The model under review builds one solid part; all positions refer to its coordinate system, in mm. A direction names the side the tool comes from. Coordinates: 2 decimals unless noted, no trailing zeros. Write each loop counter-clockwise with the first axis right and the second up, starting at its lowest first coordinate (ties: lowest second). Pieces come first, ordered by that corner, then holes. Notation, with made-up numbers: (22.5, -38.75) - (54.5, -38.75) arc R17 ccw to (54.5, -25.75) - close; hole circle Ø4 at (-4.5, -17). An arc over 180 degrees is marked (long way). Return JSON: item names as keys, results as strings. Group by question number.
(1) We need section B-B on z = 0.85. Give the number of separate pieces and of enclosed holes in the cut face, then the cut area to 3 significant figures.
(2) We need section A-A on y = 7. State the section outline as (x, z) points.
(3) To check wall thickness, follow L1, parallel to Y at x = -14, z = 0.75; L2, parallel to X at y = -26.5, z = 3.85; L3, parallel to Y at x = -42, z = 2.4. State the ranges of each line that lie inside material, in increasing order. Write a range as from..to.
(4) For pin 1 Ø2.5 at (x, z) = (-47.5, 2.5) entering from +Y; pin 2 Ø0.8 at (y, z) = (-26.5, 3.5) entering from -X; pin 3 Ø2.5 at (y, z) = (-31.5, 3) entering from +X, all flat-tipped, find the tip position at first contact; note any pin that passes through.
(5) Draft analysis for pull direction Y (two halves, no side actions). For faces 6 (the face through (50.8, 20, 3)), 7 (the face through (-1, -35.56, 3)), 8 (the face through (45.72, -10, 3)), state which applies: released by +Y, released by -Y, zero draft, split by the parting line, or undercut.
(6) Tool access review of faces 1 (the face through (48, 5.08, 3)), 2 (the face through (-45.72, 31, 3)), 3 (the face through (0, -25.146, 3)), 4 (the face through (-48, 5.08, 3)), 5 (the face through (-48, -25.4, 3)): name each direction out of +Z, -Z, +X, -X, +Y, -Y from which nothing blocks a thin tool from reaching the whole face with its end or side.
(7) We need section C-C on y = -31. State the section outline as (x, z) points, then the cut area to 3 significant figures.
Autodesk Inventor part; units mm, degrees
ref_plane "YZ Plane" through (0, 0, 0) normal (1, 0, 0) x (0, 1, 0)
ref_plane "XZ Plane" through (0, 0, 0) normal (0, 1, 0) x (-1, 0, 0)
ref_plane "XY Plane" through (0, 0, 0) normal (0, 0, 1) x (1, 0, 0)
sketch "Sketch1" plane through (0, 0, 0) normal (0, 0, 1) x (1, 0, 0)
  line L0 (-50.8, -35.56) -> (50.8, -35.56)
  line L1 (50.8, -35.56) -> (50.8, 35.56)
  line L2 (50.8, 35.56) -> (-50.8, 35.56)
  line L3 (-50.8, 35.56) -> (-50.8, -35.56)
  line L4 (-50.8, 35.56) -> (50.8, -35.56) construction
  line L5 (50.8, -35.56) -> (-50.8, -35.56) construction
  line L6 (50.8, 35.56) -> (-50.8, -35.56) construction
  point P0 (0, 0)
  point P1 (0, 0)
  dimension "d0" = 101.6
  dimension "d1" = 71.12
extrude "Extrusion1" add sketch "Sketch1" along normal blind 5.08
sketch "Sketch2" plane through (0, 0, 5.08) normal (0, 0, 1) x (1, 0, 0)
  line L0 (-43.18, 16.9024) -> (-43.18, -16.905)
  line L1 (-40.386, 16.9024) -> (-40.386, -16.905)
  line L2 (-16.9024, -27.94) -> (16.905, -27.94)
  line L3 (-16.9024, -25.146) -> (16.905, -25.146)
  line L4 (-40.386, -16.905) -> (-43.18, -16.905)
  line L5 (-43.18, 16.9024) -> (-40.386, 16.9024)
  line L6 (16.905, -25.146) -> (16.905, -27.94)
  line L7 (-16.9024, -27.94) -> (-16.9024, -25.146)
  point P0 (0, 0)
extrude "Extrusion2" cut sketch "Sketch2" against normal blind 5.08
sketch "Sketch3" plane through (0, 0, 5.08) normal (0, 0, 1) x (1, 0, 0)
  line L0 (-43.18, -16.905) -> (-43.18, 16.9024)
  line L1 (-40.386, 16.9024) -> (-40.386, -16.905)
  line L2 (16.905, -27.94) -> (-16.9024, -27.94)
  line L3 (-16.9024, -25.146) -> (16.905, -25.146)
  line L4 (50.8, -35.56) -> (50.8, 35.56)
  line L5 (50.8, 35.56) -> (-50.8, 35.56)
  line L6 (-50.8, 35.56) -> (-50.8, -35.56)
  line L7 (-50.8, -35.56) -> (50.8, -35.56)
  line L8 (50.8, -35.56) -> (50.8, 35.56)
  line L9 (50.8, 35.56) -> (45.72, 35.56)
  line L10 (45.72, 35.56) -> (45.72, 25.4)
  line L11 (45.72, 25.4) -> (50.8, 25.4)
  line L12 (50.8, 25.4) -> (50.8, 35.56)
  line L13 (0, 35.56) -> (0, -35.56) construction
  line L14 (45.72, 5.08) -> (50.8, 5.08)
  line L15 (45.72, 15.24) -> (45.72, 5.08)
  line L16 (50.8, 15.24) -> (45.72, 15.24)
  line L17 (50.8, 5.08) -> (50.8, 15.24)
  line L18 (45.72, -15.24) -> (50.8, -15.24)
  line L19 (45.72, -5.08) -> (45.72, -15.24)
  line L20 (50.8, -5.08) -> (45.72, -5.08)
  line L21 (50.8, -15.24) -> (50.8, -5.08)
  line L22 (45.72, -35.56) -> (50.8, -35.56)
  line L23 (45.72, -25.4) -> (45.72, -35.56)
  line L24 (50.8, -25.4) -> (45.72, -25.4)
  line L25 (50.8, -35.56) -> (50.8, -25.4)
  line L26 (-50.8, -35.56) -> (-50.8, 35.56)
  line L27 (-50.8, -35.56) -> (-50.8, 35.56)
  line L28 (-50.8, 35.56) -> (-45.72, 35.56)
  line L29 (-45.72, 35.56) -> (-45.72, 25.4)
  line L30 (-45.72, 25.4) -> (-50.8, 25.4)
  line L31 (-50.8, 25.4) -> (-50.8, 35.56)
  line L32 (-45.72, 5.08) -> (-50.8, 5.08)
  line L33 (-45.72, 15.24) -> (-45.72, 5.08)
  line L34 (-50.8, 15.24) -> (-45.72, 15.24)
  line L35 (-50.8, 5.08) -> (-50.8, 15.24)
  line L36 (-45.72, -15.24) -> (-50.8, -15.24)
  line L37 (-45.72, -5.08) -> (-45.72, -15.24)
  line L38 (-50.8, -5.08) -> (-45.72, -5.08)
  line L39 (-50.8, -15.24) -> (-50.8, -5.08)
  line L40 (-45.72, -35.56) -> (-50.8, -35.56)
  line L41 (-45.72, -25.4) -> (-45.72, -35.56)
  line L42 (-50.8, -25.4) -> (-45.72, -25.4)
  line L43 (-50.8, -35.56) -> (-50.8, -25.4)
  line L44 (-40.386, -16.905) -> (-43.18, -16.905)
  line L45 (-43.18, 16.9024) -> (-40.386, 16.9024)
  line L46 (16.905, -25.146) -> (16.905, -27.94)
  line L47 (-16.9024, -27.94) -> (-16.9024, -25.146)
  point P0 (0, 0)
  dimension "d6" = 10.16
  dimension "d7" = 5.08
  dimension "d8" = 0
  dimension "d11" = 20.32
  dimension "d16" = 20.32
extrude "Extrusion3" cut sketch "Sketch3" against normal blind 25.4 contours L0 L45 L1 L44 | L2 L47 L3 L46 | L24 L23 L7 L41 L42 L6 L36 L37 L38 L32 L33 L34 L30 L29 L5 L10 L11 L4 L16 L15 L14 L20 L19 L18 keep common part
sketch "Sketch4" plane through (0, 0, 5.08) normal (0, 0, 1) x (1, 0, 0)
  point P0 (0, 0)
sketch "Sketch5" plane through (0, 0, 5.08) normal (0, 0, 1) x (1, 0, 0)
  line L0 (-50.8, -15.24) -> (-45.72, -15.24)
  line L1 (-50.8, -15.24) -> (-50.8, -25.4)
  line L2 (-45.72, -25.4) -> (-50.8, -25.4)
  line L3 (-45.72, -35.56) -> (-45.72, -25.4)
  line L4 (-45.72, -35.56) -> (45.72, -35.56)
  line L5 (45.72, -25.4) -> (45.72, -35.56)
  line L6 (50.8, -25.4) -> (45.72, -25.4)
  line L7 (50.8, -25.4) -> (50.8, -15.24)
  line L8 (45.72, -15.24) -> (50.8, -15.24)
  line L9 (45.72, -5.08) -> (45.72, -15.24)
  line L10 (50.8, -5.08) -> (45.72, -5.08)
  line L11 (50.8, -5.08) -> (50.8, 5.08)
  line L12 (45.72, 5.08) -> (50.8, 5.08)
  line L13 (45.72, 15.24) -> (45.72, 5.08)
  line L14 (50.8, 15.24) -> (45.72, 15.24)
  line L15 (50.8, 15.24) -> (50.8, 25.4)
  line L16 (45.72, 25.4) -> (50.8, 25.4)
  line L17 (45.72, 35.56) -> (45.72, 25.4)
  line L18 (45.72, 35.56) -> (-45.72, 35.56)
  line L19 (-45.72, 25.4) -> (-45.72, 35.56)
  line L20 (-50.8, 25.4) -> (-45.72, 25.4)
  line L21 (-50.8, 25.4) -> (-50.8, 15.24)
  line L22 (-45.72, 15.24) -> (-50.8, 15.24)
  line L23 (-45.72, 5.08) -> (-45.72, 15.24)
  line L24 (-50.8, 5.08) -> (-45.72, 5.08)
  line L25 (-50.8, 5.08) -> (-50.8, -5.08)
  line L26 (-45.72, -5.08) -> (-50.8, -5.08)
  line L27 (-45.72, -15.24) -> (-45.72, -5.08)
  line L28 (-43.18, -16.905) -> (-43.18, 16.9024)
  line L29 (-40.386, 16.9024) -> (-40.386, -16.905)
  line L30 (16.905, -27.94) -> (-16.9024, -27.94)
  line L31 (-16.9024, -25.146) -> (16.905, -25.146)
  line L32 (-40.386, 20.0774) -> (-43.18, 20.0774)
  line L33 (-43.18, 20.0774) -> (-43.18, 14.9974)
  line L34 (-43.18, 14.9974) -> (-40.386, 14.9974)
  line L35 (-40.386, 14.9974) -> (-40.386, 20.0774)
  line L36 (-43.18, -20.08) -> (-40.386, -20.08)
  line L37 (-40.386, -20.08) -> (-40.386, -15)
  line L38 (-40.386, -15) -> (-43.18, -15)
  line L39 (-43.18, -15) -> (-43.18, -20.08)
  line L40 (-20.0774, -27.94) -> (-14.9974, -27.94)
  line L41 (-14.9974, -27.94) -> (-14.9974, -25.146)
  line L42 (-14.9974, -25.146) -> (-20.0774, -25.146)
  line L43 (-20.0774, -25.146) -> (-20.0774, -27.94)
  line L44 (20.08, -25.146) -> (15, -25.146)
  line L45 (15, -25.146) -> (15, -27.94)
  line L46 (15, -27.94) -> (20.08, -27.94)
  line L47 (20.08, -27.94) -> (20.08, -25.146)
  line L48 (-40.386, -16.905) -> (-43.18, -16.905)
  line L49 (-43.18, 16.9024) -> (-40.386, 16.9024)
  line L50 (16.905, -25.146) -> (16.905, -27.94)
  line L51 (-16.9024, -27.94) -> (-16.9024, -25.146)
  point P0 (0, 0)
  dimension "d19" = 5.08
  dimension "d20" = 5.08
  dimension "d21" = 5.08
  dimension "d22" = 5.08
extrude "Extrusion4" add sketch "Sketch5" against normal blind 5.08 contours L48 L37 L36 L39 | L28 L38 L29 L48 | L28 L49 L29 L34 | L33 L32 L35 L49 | L50 L44 L47 L46 | L30 L45 L31 L50 | L30 L51 L31 L41 | L40 L43 L42 L51
properties part number "PiShelf" material "Wood (Birch)"
Ans:
{
 "1": {"separate pieces": "1", "enclosed holes": "2", "area": "6,650 mm²"},
 "2": {"outline": "(-45.72, 0) - (-43.18, 0) - (-43.18, 5.08) - (-45.72, 5.08) - close; (-40.39, 0) - (45.72, 0) - (45.72, 5.08) - (-40.39, 5.08) - close"},
 "3": {"L1": "-35.56..-27.94, -25.15..35.56", "L2": "-45.72..-15, 15..45.72", "L3": "-35.56..-15, 15..35.56"},
 "4": {"pin 1": "y = 25.4", "pin 2": "x = -45.72", "pin 3": "x = 45.72"},
 "5": {"face 6": "zero draft", "face 7": "released by -Y", "face 8": "undercut"},
 "6": {"face 1": "+Z, -Z, +X", "face 2": "+Z, -Z, -X, +Y", "face 3": "+Z, -Z", "face 4": "+Z, -Z, -X", "face 5": "+Z, -Z, -X, -Y"},
 "7": {"outline": "(-45.72, 0) - (45.72, 0) - (45.72, 5.08) - (-45.72, 5.08) - close", "area": "465 mm²"}
}
